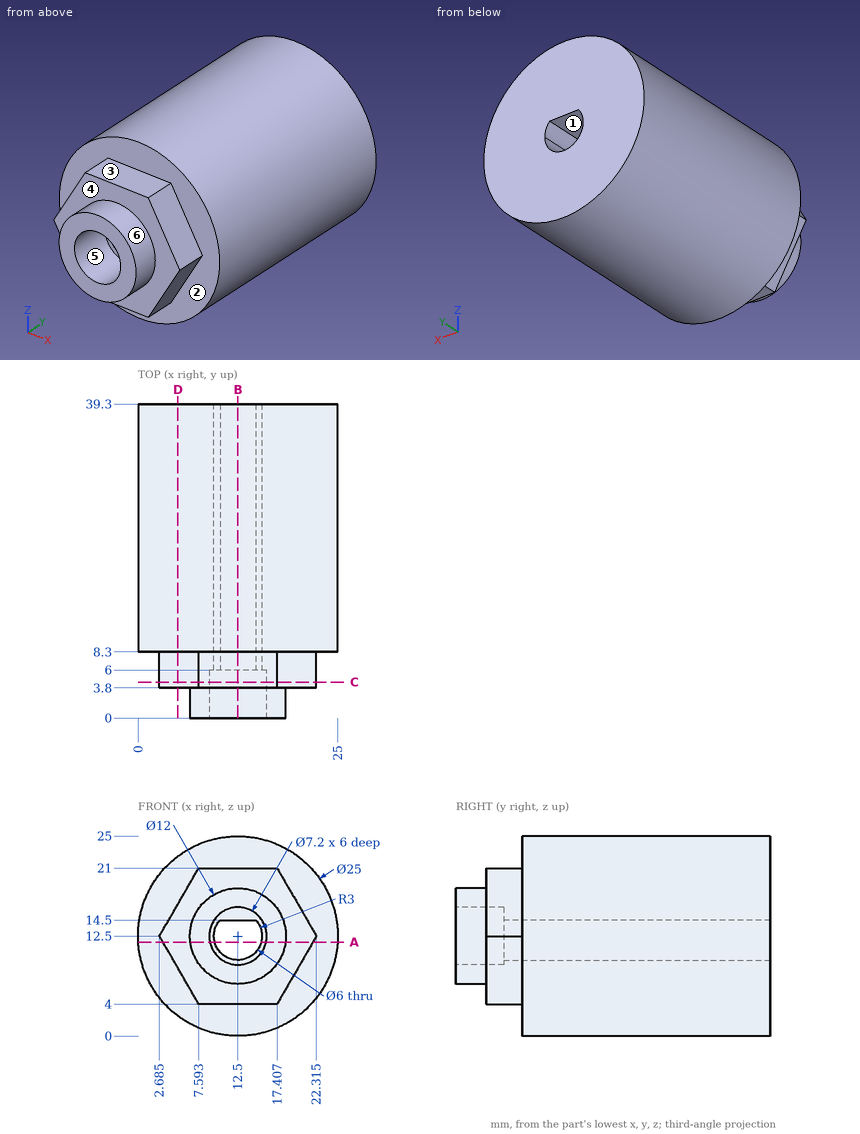
Geometry check sheet. Reference: drawing and pictorial views, mm from the part's lowest x, y, z. A direction names the side the tool comes from. Round coordinates to 2 decimals unless told otherwise and drop trailing zeros. Loops run counter-clockwise (first coordinate to the right, second up) from the corner with the lowest first, then second, coordinate; pieces in that order, holes last. Notation, with made-up numbers: (78, 65.5) -> (119, 65.5) arc R21 cw to (119, 74.5) -> close; hole circle Ø9 at (-12, 25.5). An arc over 180 degrees is marked (long way). Answer as a JSON object with one key per item and string values. Group by question number.
Item 1: Cross-section at B-B, the plane x = 12.5. Record the cut outline in (y, z).
Item 2: Cross-section at A-A, the plane z = 11.75. Record the cut outline in (x, y) (1 decimal).
Item 3: Thickness scan on line 1 along Z through (x, y) = (12.5, 4.05); line 2 along X through (y, z) = (14, 12.5); line 3 along Z through (x, y) = (12.5, 1.2). Record the ranges inside material, lowest first.
Item 4: Set-up check for the marked faces 1, 2 and 3: record each of +Z, -Z, +X, -X, +Y, -Y from which the full face is reachable in a straight line by a thin tool's end or side.
Item 5: Cross-section at C-C, the plane y = 4.5. Record the cut outline in (x, z) (1 decimal).
Item 6: Cross-section at D-D, the plane x = 5. Record the cut outline in (y, z).
Item 7: Depth check by flat-ended pin: pin 1 Ø5 at (y, z) = (26, 20.5) entering from -X (1 decimal); pin 2 Ø1 at (x, y) = (14, 30) entering from -Z; pin 3 Ø3.5 at (x, y) = (12.5, 6) entering from +Z. Enter the tip coordinate at first touch or a pass-through.
Item 8: Release check for a two-part mould opening along Z. For the marked faces 4, 5 and 6 record: pulls with the +Z half, pulls with the -Z half, needs draft (parallel to the pull), parting line crosses it, or undercut.
Determined:
{
 "1": {"outline": "(0, 6.5) -> (3.8, 6.5) -> (3.8, 4) -> (8.3, 4) -> (8.3, 0) -> (39.3, 0) -> (39.3, 9.5) -> (6, 9.5) -> (6, 8.9) -> (0, 8.9) -> close; (0, 16.1) -> (6, 16.1) -> (6, 14.5) -> (39.3, 14.5) -> (39.3, 25) -> (8.3, 25) -> (8.3, 21) -> (3.8, 21) -> (3.8, 18.5) -> (0, 18.5) -> close"},
 "2": {"outline": "(0, 8.3) -> (3.1, 8.3) -> (3.1, 3.8) -> (6.5, 3.8) -> (6.5, 0) -> (9, 0) -> (9, 6) -> (9.6, 6) -> (9.6, 39.3) -> (0, 39.3) -> close; (15.4, 6) -> (16, 6) -> (16, 0) -> (18.5, 0) -> (18.5, 3.8) -> (21.9, 3.8) -> (21.9, 8.3) -> (25, 8.3) -> (25, 39.3) -> (15.4, 39.3) -> close"},
 "3": {"line 1": "z = 4 to 8.9, 16.1 to 21", "line 2": "x = 0 to 9.5, 15.5 to 25", "line 3": "z = 6.5 to 8.9, 16.1 to 18.5"},
 "4": {"face 1": "+Y, -Y", "face 2": "-Y", "face 3": "+Z, +X, -X, -Y"},
 "5": {"outline": "(2.7, 12.5) -> (7.6, 4) -> (17.4, 4) -> (22.3, 12.5) -> (17.4, 21) -> (7.6, 21) -> close; hole circle Ø7.2 at (12.5, 12.5)"},
 "6": {"outline": "(3.8, 8.49) -> (8.3, 8.49) -> (8.3, 2.5) -> (39.3, 2.5) -> (39.3, 22.5) -> (8.3, 22.5) -> (8.3, 16.51) -> (3.8, 16.51) -> close"},
 "7": {"pin 1": "stops at x = 1.3", "pin 2": "stops at z = 0.04", "pin 3": "stops at z = 21"},
 "8": {"face 4": "needs draft", "face 5": "undercut", "face 6": "parting line crosses it"}
}
